Can you work these out from the model? Positions are in its coordinate system, mm. A direction names the side the tool comes from. Coordinates: 2 decimals unless noted, no trailing zeros. Order: outer loops, then holes, each group sorted by start corner. A loop starts at its lowest first (then second) coordinate and runs counter-clockwise, first axis right, second up. Notation, with made-up numbers: (80, 15) - (134, 15) arc R9 cw to (134, 31) - close; hole circle Ø4 at (-4.5, 24). An arc over 180 degrees is marked (long way). Return JSON: item names as keys, results as strings. Group by question number.
1) Imagine slicing it at C-C (y = -4.75). Write out the boundary of the cut face in (x, z).
2) For pin 1 Ø1.5 at (y, z) = (-1.5, 3) entering from -X; pin 2 Ø0.5 at (x, y) = (-2.5, -8) entering from +Z; pin 3 Ø1.5 at (x, y) = (4, -4.5) entering from -Z, each with a flat end and sliding along its axis, tell me the tip position at first contact or that it passes through.
3) Which directions (+Z, -Z, +X, -X, +Y, -Y) give clear straight access to the entire face, cutting with the end or side of a thin tool? Please do faces 1 (the face through (-3.81, -4, -2)), 2 (the face through (0, -4, -3.556)), 3 (the face through (0, -4, -1.016)).
4) Imagine slicing it at A-A (x = 0). Write out the boundary of the cut face in (y, z).
5) Imagine slicing it at D-D (x = -2.5). Write out the boundary of the cut face in (y, z).
6) Imagine slicing it at B-B (z = -1.25). Write out the boundary of the cut face in (x, y), and give its area (3 significant figures).
7) If I drill on line 1 along Y through (x, z) = (-1.5, 4.25); line 2 along Z through (x, y) = (-2.5, -8.75); line 3 along Z through (x, y) = (-2.5, -3.75), over which ranges is the centre line in solid material (lowest first)?
```python
from build123d import *

# Parameters (mm, degrees)
SKETCH1_R           = 6.35
BOSS_EXTRUDE1_DEPTH = 1.52
SKETCH2_W           = 7.62
SKETCH2_H           = 2.54
BOSS_EXTRUDE2_DEPTH = 4.064
SKETCH3_W           = 0.635
SKETCH3_H           = 0.635
BOSS_EXTRUDE3_DEPTH = 5.842


with BuildPart() as part:
    # Sketch1 → Boss-Extrude1 (new body)
    with BuildSketch(Plane(origin=(0, 0, 0), x_dir=(1, 0, 0), z_dir=(0, 1, 0))):
        with Locations(Location((0, 0, 0), (0, 0, 270))):
            Circle(SKETCH1_R)
    extrude(amount=-BOSS_EXTRUDE1_DEPTH)

    # Sketch2 → Boss-Extrude2 (add)
    with BuildSketch(Plane.XZ.offset(1.52)):
        with Locations((0, -2.286)):
            Rectangle(SKETCH2_W, SKETCH2_H)
    extrude(amount=BOSS_EXTRUDE2_DEPTH)

    # Sketch3 → Boss-Extrude3 (add)
    with BuildSketch(Plane.XZ.offset(5.584)):
        with Locations((0, -2.286)):
            Rectangle(SKETCH3_W, SKETCH3_H)
        with Locations((-2.54, -2.286)):
            Rectangle(SKETCH3_W, SKETCH3_H)
        with Locations((2.54, -2.286)):
            Rectangle(SKETCH3_W, SKETCH3_H)
    extrude(amount=BOSS_EXTRUDE3_DEPTH)


solid = part.part
```
Calculated:
{
 "1": {"outline": "(-3.81, -3.56) - (3.81, -3.56) - (3.81, -1.02) - (-3.81, -1.02) - close"},
 "2": {"pin 1": "x = -5.94", "pin 2": "z = -1.97", "pin 3": "z = -3.56"},
 "3": {"face 1": "+Z, -Z, -X, -Y", "face 2": "-Z, +X, -X, -Y", "face 3": "+Z, +X, -X, -Y"},
 "4": {"outline": "(-11.43, -2.6) - (-5.58, -2.6) - (-5.58, -3.56) - (-1.52, -3.56) - (-1.52, -6.35) - (0, -6.35) - (0, 6.35) - (-1.52, 6.35) - (-1.52, -1.02) - (-5.58, -1.02) - (-5.58, -1.97) - (-11.43, -1.97) - close"},
 "5": {"outline": "(-11.43, -2.6) - (-5.58, -2.6) - (-5.58, -3.56) - (-1.52, -3.56) - (-1.52, -5.84) - (0, -5.84) - (0, 5.84) - (-1.52, 5.84) - (-1.52, -1.02) - (-5.58, -1.02) - (-5.58, -1.97) - (-11.43, -1.97) - close"},
 "6": {"outline": "(-6.23, -1.52) - (-3.81, -1.52) - (-3.81, -5.58) - (3.81, -5.58) - (3.81, -1.52) - (6.23, -1.52) - (6.23, 0) - (-6.23, 0) - close", "area": "49.9 mm2"},
 "7": {"line 1": "-1.52 to 0", "line 2": "-2.6 to -1.97", "line 3": "-3.56 to -1.02"}
}
